from build123d import *

# Parameters (mm, degrees)
F0_W      = 330
F0_H      = 390
F1_DEPTH  = 7
F2_R      = 1.5
F3_DEPTH  = 25
F4_R      = 1.5
F5_DEPTH  = 25
F7_DEPTH  = 5
F9_DEPTH  = 25
F10_R     = 5
F11_DEPTH = 25
F12_R     = 1
F13_DEPTH = 50
F14_R     = 1
F15_DEPTH = 5


with BuildPart() as f1:
    # F0 (on Top) → F1 (new body)
    with BuildSketch(Plane.XY):
        Rectangle(F0_W, F0_H)
    extrude(amount=F1_DEPTH)

    # F2 (on face) → F3 (cut)
    with BuildSketch(Plane.XY.offset(7)):
        with Locations((-155, 40)):
            Circle(F2_R)
        with Locations((-155, -40)):
            Circle(F2_R)
    extrude(amount=-F3_DEPTH, mode=Mode.SUBTRACT)

    # F4 (on face) → F5 (cut)
    with BuildSketch(Plane.XY.offset(7)):
        with Locations((155, 40)):
            Circle(F4_R)
        with Locations((155, -40)):
            Circle(F4_R)
    extrude(amount=-F5_DEPTH, mode=Mode.SUBTRACT)

    # F6 (on face) → F7 (cut)
    with BuildSketch(Plane.XY.offset(7)):
        with BuildLine():
            Line((-138, 56.771628), (-137, 56.771628))
            ThreePointArc((-137, 56.771628), (-138.707107, 57.478734), (-138, 55.771628))
            Line((-138, 55.771628), (-138, 56.771628))
        make_face()
        with BuildLine():
            ThreePointArc((-136.845755, 16.771628), (-137.195464, 17.531314), (-138, 17.75966))
            Line((-138, 17.75966), (-138, 16.771628))
            Line((-138, 16.771628), (-138.845755, 16.771628))
            ThreePointArc((-138.845755, 16.771628), (-137.845755, 15.771628), (-136.845755, 16.771628))
        make_face()
        with BuildLine():
            Line((-138, 16.771628), (-138, 17.75966))
            ThreePointArc((-138, 17.75966), (-138.605441, 17.421918), (-138.845755, 16.771628))
            Line((-138.845755, 16.771628), (-138, 16.771628))
        make_face()
        with BuildLine():
            ThreePointArc((-138, 55.771628), (-137.292893, 56.064521), (-137, 56.771628))
            Line((-137, 56.771628), (-138, 56.771628))
            Line((-138, 56.771628), (-138, 55.771628))
        make_face()
        with BuildLine():
            ThreePointArc((-82, 56.771628), (-83, 57.771628), (-84, 56.771628))
            ThreePointArc((-84, 56.771628), (-83, 55.771628), (-82, 56.771628))
        make_face()
    extrude(amount=-F7_DEPTH, mode=Mode.SUBTRACT)

    # F8 (on face) → F9 (cut)
    with BuildSketch(Plane.XY.offset(7)):
        Polygon((-145, 7.5), (-145, 0), (-145, -7.5), (-85, -7.5), (-85, 7.5), align=None)
    extrude(amount=-F9_DEPTH, mode=Mode.SUBTRACT)

    # F10 (on face) → F11 (cut)
    with BuildSketch(Plane.XY.offset(7)):
        Circle(F10_R)
    extrude(amount=-F11_DEPTH, mode=Mode.SUBTRACT)

    # F12 (on face) → F13 (cut)
    with BuildSketch(Plane.XY.offset(7)):
        with Locations((10, 185)):
            Circle(F12_R)
        with Locations((-10, 185)):
            Circle(F12_R)
        with Locations((10, -185)):
            Circle(F12_R)
        with Locations((-10, -185)):
            Circle(F12_R)
    extrude(amount=-F13_DEPTH, mode=Mode.SUBTRACT)

    # F14 (on face) → F15 (cut)
    with BuildSketch(Plane(origin=(0, 0, 0), x_dir=(1, 0, 0), z_dir=(0, 0, -1))):
        with Locations((10, 140)):
            Circle(F14_R)
    extrude(amount=-F15_DEPTH, mode=Mode.SUBTRACT)


solid = f1.part
Source: CAD feature listing. Evaluate the final solid. Frame: model axes, mm. Give positions to 0.01 mm unless a question says otherwise; leave off trailing zeros. Use a Markdown table: item, result.
1) Ray query, line 1 along Y through (x, z) = (-10, 3.75); line 2 along Y through (x, z) = (155, 5); line 3 along X through (y, z) = (-140, 1.9). Return the intervals inside material, ascending. Write a range as [from, to].
Answer list:
| item | result |
|---|---|
| line 1 | [-195, -186], [-184, 184], [186, 195] |
| line 2 | [-195, -41.5], [-38.5, 38.5], [41.5, 195] |
| line 3 | [-165, 9], [11, 165] |
2) Contact query for flat-ended pins moving along their axis: P1, Ø1.8, axis at x = 155, y = 40, coming from the -Z side; P2, Ø1, axis at x = -83, y = 56.5, coming from the +Z side. Output: stop coordinate, or through.
Answer list:
| item | result |
|---|---|
| P1 | through |
| P2 | z = 2 |
3) Mould query, pull axis Y, two halves, no side actions, for faces 1 (the flat face through (34, 3, 0)), 2 (the cylindrical face through (-1.08, -4.88, 3.55)). Classes: +Y half, -Y half, draft (parallel to the pull), parting line (faces both ways), or undercut.
Answer list:
| item | result |
|---|---|
| face 1 | draft |
| face 2 | undercut |
